Work out the finished part from the listing and answer in its coordinate system (mm). Give positions to 0.01 mm unless a question says otherwise; leave off trailing zeros. Loops run counter-clockwise (first coordinate to the right, second up) from the corner with the lowest first, then second, coordinate; pieces in that order, holes last. Notation, with made-up numbers: M 42,54 L 91,54 A20 cw 91,83 Z; hole C -30.5,-23 d10. An arc over 180 degrees is marked long. Answer in a Markdown table with one row per item. Add a question column.
from build123d import *

# Parameters (mm, degrees)
SKETCH1_W                                = 49.8
SKETCH1_H                                = 39.8
BOSS_EXTRUDE1_DEPTH                      = 3
CUT_EXTRUDE1_DEPTH                       = 3
MIRROR1_AT_THE_SECOND_PLANE_COPY_1_DEPTH = 3
SKETCH3_W                                = 35.8
SKETCH3_H                                = 27.8
CUT_EXTRUDE2_DEPTH                       = 3
SKETCH4_W                                = 57.8
SKETCH4_H                                = 47.8
SKETCH4_W_2                              = 49.8
SKETCH4_H_2                              = 39.8
BOSS_EXTRUDE2_DEPTH                      = 3


with BuildPart() as part:
    # Sketch1 → Boss-Extrude1 (new body)
    with BuildSketch(Plane(origin=(0, 0, 0), x_dir=(1, 0, 0), z_dir=(0, 1, 0))):
        Rectangle(SKETCH1_W, SKETCH1_H)
    extrude(amount=BOSS_EXTRUDE1_DEPTH)

    # Sketch2 → Cut-Extrude1 (cut)
    with BuildSketch(Plane(origin=(0, 3, 0), x_dir=(1, 0, 0), z_dir=(0, 1, 0))):
        with BuildLine():
            ThreePointArc((-21.9, 14.4), (-20.132233047, 15.132233047), (-19.4, 16.9))
            Line((-19.4, 16.9), (-21.9, 16.9))
            Line((-21.9, 16.9), (-21.9, 14.4))
        make_face()
        with BuildLine():
            Line((-21.9, 16.9), (-19.4, 16.9))
            ThreePointArc((-19.4, 16.9), (-23.667766953, 18.667766953), (-21.9, 14.4))
            Line((-21.9, 14.4), (-21.9, 16.9))
        make_face()
    cut_extrude1 = extrude(amount=-CUT_EXTRUDE1_DEPTH, mode=Mode.SUBTRACT)

    # Mirror1: Cut-Extrude1 across plane
    add(cut_extrude1.mirror(Plane(origin=(0, 0, 0), x_dir=(0, 0, 1), z_dir=(1, 0, 0))), mode=Mode.SUBTRACT)

    # Mirror1 at the second plane: Cut-Extrude1 across plane
    add(cut_extrude1.mirror(Plane(origin=(0, 0, 0), x_dir=(1, 0, 0), z_dir=(0, 0, -1))), mode=Mode.SUBTRACT)

    # Mirror1 at the second plane copy 1 sketc → Mirror1 at the second plane copy 1 (cut)
    with BuildSketch(Plane(origin=(0, 3, 0), x_dir=(-1, 0, 0), z_dir=(0, 1, 0))):
        with BuildLine():
            ThreePointArc((-21.9, 14.4), (-20.132233047, 15.132233047), (-19.4, 16.9))
            Line((-19.4, 16.9), (-21.9, 16.9))
            Line((-21.9, 16.9), (-21.9, 14.4))
        make_face()
        with BuildLine():
            Line((-21.9, 16.9), (-19.4, 16.9))
            ThreePointArc((-19.4, 16.9), (-23.667766953, 18.667766953), (-21.9, 14.4))
            Line((-21.9, 14.4), (-21.9, 16.9))
        make_face()
    extrude(amount=-MIRROR1_AT_THE_SECOND_PLANE_COPY_1_DEPTH, mode=Mode.SUBTRACT)

    # Sketch3 → Cut-Extrude2 (cut)
    with BuildSketch(Plane(origin=(0, 3, 0), x_dir=(1, 0, 0), z_dir=(0, 1, 0))):
        Rectangle(SKETCH3_W, SKETCH3_H)
    extrude(amount=-CUT_EXTRUDE2_DEPTH, mode=Mode.SUBTRACT)

    # Sketch4 → Boss-Extrude2 (add)
    with BuildSketch(Plane(origin=(0, 3, 0), x_dir=(1, 0, 0), z_dir=(0, 1, 0))):
        Rectangle(SKETCH4_W, SKETCH4_H)
        Rectangle(SKETCH4_W_2, SKETCH4_H_2, mode=Mode.SUBTRACT)
    extrude(amount=-BOSS_EXTRUDE2_DEPTH)


solid = part.part
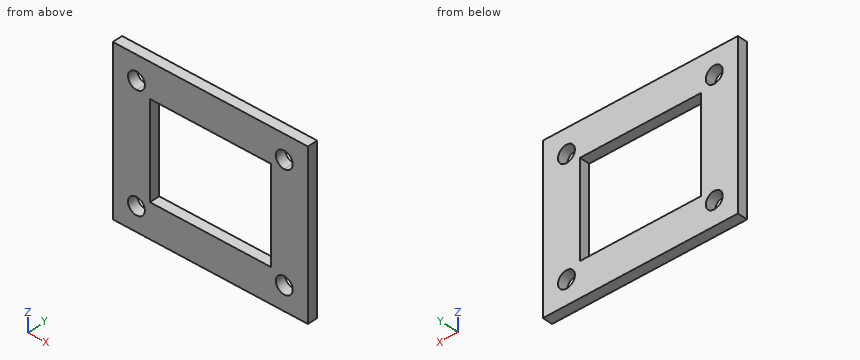
(1) Consider line 1 along X through (y, z) = (1.25, -16.9); line 2 along Z through (x, y) = (-21.9, 1.9); line 3 along Z through (x, y) = (-10.5, 0.95). Determine where each line is inside the solid, lowest interval first. Write a range as from..to.
(2) Each of these flat-tipped pins is pushed along its axis until it touches: P1, Ø8, axis at x = 21.9, z = 16.9, coming from the -Y side; P2, Ø4.5, axis at x = -21.9, z = -16.9, coming from the +Y side. Where does it stop, or does it pass through?
(3) Section A-A, the plane x = 7 is taken. Determine the outline of the cut face in (y, z).
(4) Section D-D, the plane x = -20.5 is taken. Determine the outline of the cut face in (y, z), and give its area (3 significant figures).
(5) Section C-C, the plane z = -10.5 is taken. Determine the outline of the cut face in (x, y).
(6) Section B-B, the plane y = 1.35 is taken. Determine the outline of the cut face in (x, z).
Numbers:
| question | item | result |
|---|---|---|
| 1 | line 1 | x = -28.9..-24.4, -19.4..19.4, 24.4..28.9 |
| 1 | line 2 | z = -23.9..-19.4, -14.4..14.4, 19.4..23.9 |
| 1 | line 3 | z = -23.9..-13.9, 13.9..23.9 |
| 2 | P1 | stops at y = 0 |
| 2 | P2 | passes through |
| 3 | outline | M 0,-23.9 L 3,-23.9 L 3,-13.9 L 0,-13.9 Z; M 0,13.9 L 3,13.9 L 3,23.9 L 0,23.9 Z |
| 4 | outline | M 0,-23.9 L 3,-23.9 L 3,-18.97 L 0,-18.97 Z; M 0,-14.83 L 3,-14.83 L 3,14.83 L 0,14.83 Z; M 0,18.97 L 3,18.97 L 3,23.9 L 0,23.9 Z |
| 4 | area | 119 mm² |
| 5 | outline | M -28.9,0 L -17.9,0 L -17.9,3 L -28.9,3 Z; M 17.9,0 L 28.9,0 L 28.9,3 L 17.9,3 Z |
| 6 | outline | M -28.9,-23.9 L 28.9,-23.9 L 28.9,23.9 L -28.9,23.9 Z; hole C -21.9,-16.9 d5; hole C -21.9,16.9 d5; hole M -17.9,-13.9 L 17.9,-13.9 L 17.9,13.9 L -17.9,13.9 Z; hole C 21.9,-16.9 d5; hole C 21.9,16.9 d5 |
